Autodesk Inventor part; units mm, degrees
ref_plane "YZ Plane" through (0, 0, 0) normal (1, 0, 0) x (0, 1, 0)
ref_plane "XZ Plane" through (0, 0, 0) normal (0, 1, 0) x (-1, 0, 0)
ref_plane "XY Plane" through (0, 0, 0) normal (0, 0, 1) x (1, 0, 0)
sketch "Sketch5" plane through (0, 0, 0) normal (0, 0, 1) x (1, 0, 0)
  circle A0 centre (-16, 16) radius 1.75
  line L0 (-3.5516, 0) -> (2.966, 0)
  line L1 (0, 4.5757) -> (0, -5.4514)
  circle A1 centre (16, 16) radius 1.75
  circle A2 centre (-16, -16) radius 1.75
  circle A3 centre (16, -16) radius 1.75
  line L2 (19, -19) -> (-19, -19)
  line L3 (-19, -19) -> (-19, 19)
  line L4 (-19, 19) -> (19, 19)
  line L5 (19, 19) -> (19, -19)
  line L6 (19, -19) -> (-19, 19) construction
  line L7 (-19, -19) -> (19, 19) construction
  line L8 (4.0992, -12.7) -> (2.0496, -16.25)
  line L9 (2.0496, -16.25) -> (-2.0496, -16.25)
  line L10 (-2.0496, -16.25) -> (-4.0992, -12.7)
  line L11 (-4.0992, -12.7) -> (-2.0496, -9.15)
  line L12 (-2.0496, -9.15) -> (2.0496, -9.15)
  line L13 (2.0496, -9.15) -> (4.0992, -12.7)
  line L14 (4.0992, 12.7) -> (2.0496, 9.15)
  line L15 (2.0496, 9.15) -> (-2.0496, 9.15)
  line L16 (-2.0496, 9.15) -> (-4.0992, 12.7)
  line L17 (-4.0992, 12.7) -> (-2.0496, 16.25)
  line L18 (-2.0496, 16.25) -> (2.0496, 16.25)
  line L19 (2.0496, 16.25) -> (4.0992, 12.7)
  point P0 (0, 0)
  point P1 (0, 12.7)
  point P2 (0, -12.7)
  point P3 (0, -12.7)
  point P4 (0, 12.7)
  point P5 (0, -16.25)
  dimension "d47" = 3.5
  dimension "d50" = 32
  dimension "d53" = 32
  dimension "d56" = 16
  dimension "d57" = 16
  dimension "d58" = 38
  dimension "d59" = 38
  dimension "d73" = 7.1
  dimension "d74" = 7.1
extrude "Extrusion3" add sketch "Sketch5" along normal blind 5 contours L2 L3 L4 L5 | L8 L9 L10 L11 L12 L13 | L14 L15 L16 L17 L18 L19
sketch "Sketch6" plane through (0, 0, 5) normal (0, 0, 1) x (1, 0, 0)
  circle A0 centre (-16, 16) radius 1.75
  line L0 (-16, 19.4641) -> (-13, 17.7321)
  line L1 (-13, 17.7321) -> (-13, 14.2679)
  line L2 (-13, 14.2679) -> (-16, 12.5359)
  line L3 (-16, 12.5359) -> (-19, 14.2679)
  line L4 (-19, 14.2679) -> (-19, 17.7321)
  line L5 (-19, 17.7321) -> (-16, 19.4641)
  line L6 (0, 4.5757) -> (0, -5.4514)
  line L7 (-3.5516, 0) -> (2.966, 0)
  line L8 (16, 19.4641) -> (19, 17.7321)
  line L9 (19, 17.7321) -> (19, 14.2679)
  line L10 (19, 14.2679) -> (16, 12.5359)
  line L11 (16, 12.5359) -> (13, 14.2679)
  line L12 (13, 14.2679) -> (13, 17.7321)
  line L13 (13, 17.7321) -> (16, 19.4641)
  line L14 (-16, -12.5359) -> (-13, -14.2679)
  line L15 (-13, -14.2679) -> (-13, -17.7321)
  line L16 (-13, -17.7321) -> (-16, -19.4641)
  line L17 (-16, -19.4641) -> (-19, -17.7321)
  line L18 (-19, -17.7321) -> (-19, -14.2679)
  line L19 (-19, -14.2679) -> (-16, -12.5359)
  line L20 (16, -12.5359) -> (19, -14.2679)
  line L21 (19, -14.2679) -> (19, -17.7321)
  line L22 (19, -17.7321) -> (16, -19.4641)
  line L23 (16, -19.4641) -> (13, -17.7321)
  line L24 (13, -17.7321) -> (13, -14.2679)
  line L25 (13, -14.2679) -> (16, -12.5359)
  point P0 (0, 0)
  point P1 (-13, 16)
  point P2 (16, 16)
  point P3 (16, 16)
  point P4 (19, 16)
  point P5 (-16, -16)
  point P6 (-16, -16)
  point P7 (-13, -16)
  point P8 (16, -16)
  point P9 (16, -16)
  point P10 (19, -16)
  dimension "d62" = 6
  dimension "d65" = 32
  dimension "d68" = 32
extrude "Extrusion4" cut sketch "Sketch6" against normal blind 2.5
hole "Hole4" at (0, 12.7, 0) at (0, -12.7, 0) direction (0, 0, 1) diameter 4.2 end through all
sketch "Sketch7" plane through (0, 0, 5) normal (0, 0, 1) x (1, 0, 0)
  line L0 (-16.8038, -19) -> (-19, -17.7321)
  line L1 (-19, -19) -> (-19, 19)
  line L2 (19, -19) -> (-19, -19)
  line L3 (19, -19) -> (-19, 19) construction
  line L4 (-19, 17.7321) -> (-16.8038, 19)
  line L5 (-19, 19) -> (19, 19)
  line L6 (16.8038, 19) -> (19, 17.7321)
  line L7 (19, 19) -> (19, -19)
  line L8 (19, -17.7321) -> (16.8038, -19)
  point P0 (0, 0)
extrude "Extrusion6" cut sketch "Sketch7" against normal up to surface (2.5 mm away) contours L2 L1 L0 | L8 L7 L2 | L1 L5 L4 | L6 L5 L7
sketch "Sketch8" plane through (0, 0, 5) normal (0, 0, 1) x (1, 0, 0)
  line L0 (15.1962, 19) -> (-15.1962, 19)
  line L1 (12.5, -19) -> (-12.5, -19)
  line L2 (-12.5, -19) -> (-12.5, 19)
  line L3 (-12.5, 19) -> (12.5, 19)
  line L4 (12.5, 19) -> (12.5, -19)
  line L5 (12.5, -19) -> (-12.5, 19) construction
  line L6 (-12.5, -19) -> (12.5, 19) construction
  circle A0 centre (0, 12.7) radius 2.1
  circle A1 centre (0, -12.7) radius 2.1
  point P0 (0, 0)
  dimension "d86" = 25
extrude "Extrusion7" add sketch "Sketch8" along normal blind 10
hole "Hole5" at (0, -12.7, 0) at (0, 12.7, 0) direction (0, 0, 1) diameter 8 depth 8
properties part number "RD-PDT-S-to-M4-bolts"
Read the model definition and answer for the solid it produces. Units are mm, in the model's axes. A direction names the side the tool comes from. Coordinates: 2 decimals unless noted, no trailing zeros. Loops run counter-clockwise (first coordinate to the right, second up) from the corner with the lowest first, then second, coordinate; pieces in that order, holes last. Notation, with made-up numbers: (57.25, 10) - (63.25, 10) arc R34 cw to (63.25, 47) - close; hole circle Ø10 at (27.25, -36.5). An arc over 180 degrees is marked (long way). Answer in a Markdown table with one row per item.
Q1. Find section B-B on x = 0. Write down the section's boundary in (y, z).
Here are the results:
| item | result |
|---|---|
| outline | (-19, 0) - (-16.7, 0) - (-16.7, 8) - (-14.8, 8) - (-14.8, 15) - (-19, 15) - close; (-10.6, 8) - (-8.7, 8) - (-8.7, 0) - (8.7, 0) - (8.7, 8) - (10.6, 8) - (10.6, 15) - (-10.6, 15) - close; (14.8, 8) - (16.7, 8) - (16.7, 0) - (19, 0) - (19, 15) - (14.8, 15) - close |
Q2. Straight lines are drawn through the part: line 1 along Y through (x, z) = (16, 2); line 2 along Y through (x, z) = (-3, 3.75); line 3 along X through (y, z) = (12.7, 4.25). For each, find the intervals that lie inside material, in ascending order. Write a range as [from, to].
Here are the results:
| item | result |
|---|---|
| line 1 | y = [-19, -17.75], [-14.25, 14.25], [17.75, 19] |
| line 2 | y = [-19, -15.35], [-10.05, 10.05], [15.35, 19] |
| line 3 | x = [-19, -16.28], [-15.72, -4], [4, 15.72], [16.28, 19] |
Q3. Find section A-A on z = 11.5. Write down the section's boundary in (x, y).
Here are the results:
| item | result |
|---|---|
| outline | (-12.5, -19) - (12.5, -19) - (12.5, 19) - (-12.5, 19) - close; hole circle Ø4.2 at (0, -12.7); hole circle Ø4.2 at (0, 12.7) |
Q4. The mould has two halves that part along Y. Classify faces 5 (the flat face through (0, 19, 7)), 6 (the cylindrical face through (-0.46, 14.75, 11.45)), 7 (the cylindrical face through (-0.176, -16.696, 4.056)), 8 (the flat face through (12.5, 0, 10)): pulls with the +Y half, pulls with the -Y half, needs draft (parallel to the pull), parting line crosses it, or undercut.
Here are the results:
| item | result |
|---|---|
| face 5 | pulls with the +Y half |
| face 6 | undercut |
| face 7 | undercut |
| face 8 | needs draft |
Q5. Find section D-D on y = -4. Write down the section's boundary in (x, z).
Here are the results:
| item | result |
|---|---|
| outline | (-19, 0) - (19, 0) - (19, 5) - (12.5, 5) - (12.5, 15) - (-12.5, 15) - (-12.5, 5) - (-19, 5) - close |
Q6. For faces 1 (the flat face through (14.113, -18.375, 3.768)), 2 (the flat face through (16, 0, 5)), 3 (the flat face through (-14.113, 18.375, 3.768)), 4 (the flat face through (-16, 0, 5)), determine the directions among +Z, -Z, +X, -X, +Y, -Y from which every point of the face is accessible in a straight line to the end or side of a thin tool.
Here are the results:
| item | result |
|---|---|
| face 1 | +Z, +X |
| face 2 | +Z, +X, +Y, -Y |
| face 3 | +Z, -X |
| face 4 | +Z, -X, +Y, -Y |
Q7. Find section C-C on y = 16. Write down the section's boundary in (x, z), plus the area to 3 significant figures.
Here are the results:
| item | result |
|---|---|
| outline | (-19, 0) - (-17.75, 0) - (-17.75, 2.5) - (-19, 2.5) - close; (-14.25, 0) - (-2.26, 0) - (-2.26, 8) - (2.26, 8) - (2.26, 0) - (14.25, 0) - (14.25, 2.5) - (13, 2.5) - (13, 5) - (12.5, 5) - (12.5, 15) - (-12.5, 15) - (-12.5, 5) - (-13, 5) - (-13, 2.5) - (-14.25, 2.5) - close; (17.75, 0) - (19, 0) - (19, 2.5) - (17.75, 2.5) - close |
| area | 356 mm^2 |
Q8. Given P1, Ø0.8, axis at y = 15.5, z = 3.5, coming from the +X side; P2, Ø2, axis at y = -16, z = 4, coming from the -X side; P3, Ø4, axis at x = 1, y = 12, coming from the -Z side, each flat-ended and moving along its own axis, determine where each tip first touches the part or whether it passes through.
Here are the results:
| item | result |
|---|---|
| P1 | stops at x = 13 |
| P2 | stops at x = -13 |
| P3 | stops at z = 8 |
